For this review, take the finished solid that the model builds, in its own axes (mm). A direction names the side the tool comes from. Coordinates: 2 decimals unless noted, no trailing zeros. Write each loop counter-clockwise with the first axis right and the second up, starting at its lowest first coordinate (ties: lowest second). Pieces come first, ordered by that corner, then holes.
1) We need section A-A on z = 9.25. Write out the cut boundary in (x, y), then the cut area to 3 significant figures.
2) We need section B-B on y = -26.5. Write out the cut boundary in (x, z), then the cut area to 3 significant figures.
3) Mouldability with a two-part tool opening along Y and no side actions: class faces 3 (the face through (37, 55, 15)), 4 (the face through (42, 72.633, 12)), 5 (the face through (41, -66.524, 12)) as pulls with the +Y half, pulls with the -Y half, needs draft (parallel to the pull), parting line crosses it, or undercut.
4) To check wall thickness, follow line 1 along Y through (x, z) = (37, 18.5) (3 decimals); line 2 along Y through (x, z) = (32.5, 18.5); line 3 along Z through (x, y) = (31.5, -34). State the ranges of each line that lie inside material, in increasing order.
5) We need section C-C on x = 39. Write out the cut boundary in (y, z), then the cut area to 3 significant figures.
6) For faces 1 (the face through (32, -31, 3)), 2 (the face through (54.099, 2, 12)), list the 3-axis set-ups (+Z, -Z, +X, -X, +Y, -Y) from which the entire face can be reached by the end or side of a thin tool; tool diameter is ignored.
7) Insertion check: P1, Ø7, axis at x = 33.5, y = 52, coming from the +Z side; P2, Ø3, axis at x = 32.5, y = -28, coming from the +Z side. Each pin has a flat end and moves straight along its axis. Give the tip position at first contact, or say it passes through.
8) We need section D-D on z = 19.25. Write out the cut boundary in (x, y).
from build123d import *

# Parameters (mm, degrees)
F1_DEPTH = 25
F2_DEPTH = 3
F3_DEPTH = 15
F4_W     = 25
F4_H     = 139.1576522589
F5_DEPTH = 3


with BuildPart() as f1:
    # F0 (on Top) → F1 (new body)
    with BuildSketch(Plane.XY):
        with BuildLine():
            Line((54.0989699066, 72.6331850421), (29.0989699066, 72.6331850421))
            Line((29.0989699066, 72.6331850421), (29.0989699066, 67.49929167))
            ThreePointArc((29.0989699066, 67.49929167), (37.8737569223, 63.8034575596), (41.5, 54.9996834778))
            ThreePointArc((41.5, 54.9996834778), (37.8737569223, 46.195909396), (29.0989699066, 42.5000752856))
            Line((29.0989699066, 42.5000752856), (29.0989699066, 39.5786203772))
            ThreePointArc((29.0989699066, 39.5786203772), (37.8737569223, 35.8827862669), (41.5, 27.079012185))
            ThreePointArc((41.5, 27.079012185), (37.8737569223, 18.2752381032), (29.0989699066, 14.5794039929))
            Line((29.0989699066, 14.5794039929), (29.0989699066, 10.4122504635))
            ThreePointArc((29.0989699066, 10.4122504635), (37.8737569223, 6.7164163532), (41.5, -2.0873577287))
            ThreePointArc((41.5, -2.0873577287), (37.8737569223, -10.8911318105), (29.0989699066, -14.5869659208))
            Line((29.0989699066, -14.5869659208), (29.0989699066, -18.4864327763))
            ThreePointArc((29.0989699066, -18.4864327763), (37.8737569223, -22.1822668866), (41.5, -30.9860409684))
            ThreePointArc((41.5, -30.9860409684), (37.8737569223, -39.7898150502), (29.0989699066, -43.4856491606))
            Line((29.0989699066, -43.4856491606), (29.0989699066, -66.5244672167))
            Line((29.0989699066, -66.5244672167), (54.0989699066, -66.5244672167))
            Line((54.0989699066, -66.5244672167), (54.0989699066, 72.6331850421))
        make_face()
    extrude(amount=F1_DEPTH)



with BuildPart() as f2:
    # F0 (on Top) → F2 (new body)
    with BuildSketch(Plane.XY):
        with BuildLine():
            ThreePointArc((35.5, 54.9996834778), (33.6310530332, 59.5607521907), (29.0989699066, 61.4989299693))
            Line((29.0989699066, 61.4989299693), (29.0989699066, 48.5004369863))
            ThreePointArc((29.0989699066, 48.5004369863), (33.6310530332, 50.4386147649), (35.5, 54.9996834778))
        make_face()
    extrude(amount=F2_DEPTH)


with BuildPart() as f2b:
    # F0 (on Top) → F2, piece 2 (new body)
    with BuildSketch(Plane.XY):
        with BuildLine():
            ThreePointArc((35.5, 27.079012185), (33.6310530332, 31.6400808979), (29.0989699066, 33.5782586765))
            Line((29.0989699066, 33.5782586765), (29.0989699066, 20.5797656935))
            ThreePointArc((29.0989699066, 20.5797656935), (33.6310530332, 22.5179434721), (35.5, 27.079012185))
        make_face()
    extrude(amount=F2_DEPTH)


with BuildPart() as f2c:
    # F0 (on Top) → F2, piece 3 (new body)
    with BuildSketch(Plane.XY):
        with BuildLine():
            Line((29.0989699066, 4.4118887628), (29.0989699066, -8.5866042202))
            ThreePointArc((29.0989699066, -8.5866042202), (33.6310530332, -6.6484264416), (35.5, -2.0873577287))
            ThreePointArc((35.5, -2.0873577287), (33.6310530332, 2.4737109842), (29.0989699066, 4.4118887628))
        make_face()
    extrude(amount=F2_DEPTH)


with BuildPart() as f2d:
    # F0 (on Top) → F2, piece 4 (new body)
    with BuildSketch(Plane.XY):
        with BuildLine():
            Line((29.0989699066, -24.4867944769), (29.0989699066, -37.4852874599))
            ThreePointArc((29.0989699066, -37.4852874599), (33.6310530332, -35.5471096813), (35.5, -30.9860409684))
            ThreePointArc((35.5, -30.9860409684), (33.6310530332, -26.4249722555), (29.0989699066, -24.4867944769))
        make_face()
    extrude(amount=F2_DEPTH)


with BuildPart() as f1_1:
    add(f1.part)

    add(f2.part)  # F3 merges F2

    add(f2b.part)  # F3 merges F2b

    add(f2c.part)  # F3 merges F2c

    add(f2d.part)  # F3 merges F2d
    # F0 (on Top) → F3 (join)
    with BuildSketch(Plane.XY):
        with BuildLine():
            ThreePointArc((41.5, 54.9996834778), (37.8737569223, 63.8034575596), (29.0989699066, 67.49929167))
            Line((29.0989699066, 67.49929167), (29.0989699066, 61.4989299693))
            ThreePointArc((29.0989699066, 61.4989299693), (33.6310530332, 59.5607521907), (35.5, 54.9996834778))
            ThreePointArc((35.5, 54.9996834778), (33.6310530332, 50.4386147649), (29.0989699066, 48.5004369863))
            Line((29.0989699066, 48.5004369863), (29.0989699066, 42.5000752856))
            ThreePointArc((29.0989699066, 42.5000752856), (37.8737569223, 46.195909396), (41.5, 54.9996834778))
        make_face()
        with BuildLine():
            ThreePointArc((41.5, 27.079012185), (37.8737569223, 35.8827862669), (29.0989699066, 39.5786203772))
            Line((29.0989699066, 39.5786203772), (29.0989699066, 33.5782586765))
            ThreePointArc((29.0989699066, 33.5782586765), (33.6310530332, 31.6400808979), (35.5, 27.079012185))
            ThreePointArc((35.5, 27.079012185), (33.6310530332, 22.5179434721), (29.0989699066, 20.5797656935))
            Line((29.0989699066, 20.5797656935), (29.0989699066, 14.5794039929))
            ThreePointArc((29.0989699066, 14.5794039929), (37.8737569223, 18.2752381032), (41.5, 27.079012185))
        make_face()
        with BuildLine():
            Line((29.0989699066, -8.5866042202), (29.0989699066, -14.5869659208))
            ThreePointArc((29.0989699066, -14.5869659208), (37.8737569223, -10.8911318105), (41.5, -2.0873577287))
            ThreePointArc((41.5, -2.0873577287), (37.8737569223, 6.7164163532), (29.0989699066, 10.4122504635))
            Line((29.0989699066, 10.4122504635), (29.0989699066, 4.4118887628))
            ThreePointArc((29.0989699066, 4.4118887628), (33.6310530332, 2.4737109842), (35.5, -2.0873577287))
            ThreePointArc((35.5, -2.0873577287), (33.6310530332, -6.6484264416), (29.0989699066, -8.5866042202))
        make_face()
        with BuildLine():
            Line((29.0989699066, -37.4852874599), (29.0989699066, -43.4856491606))
            ThreePointArc((29.0989699066, -43.4856491606), (37.8737569223, -39.7898150502), (41.5, -30.9860409684))
            ThreePointArc((41.5, -30.9860409684), (37.8737569223, -22.1822668866), (29.0989699066, -18.4864327763))
            Line((29.0989699066, -18.4864327763), (29.0989699066, -24.4867944769))
            ThreePointArc((29.0989699066, -24.4867944769), (33.6310530332, -26.4249722555), (35.5, -30.9860409684))
            ThreePointArc((35.5, -30.9860409684), (33.6310530332, -35.5471096813), (29.0989699066, -37.4852874599))
        make_face()
    extrude(amount=F3_DEPTH)

    # F4 (on face) → F5 (join)
    with BuildSketch(Plane(origin=(0, 0, 0), x_dir=(1, 0, 0), z_dir=(0, 0, -1))):
        with Locations((41.5989699066, -3.0543589127)):
            Rectangle(F4_W, F4_H)
    extrude(amount=-F5_DEPTH)


solid = f1_1.part
Result:
1. outline: (29.1, -66.52) - (54.1, -66.52) - (54.1, 72.63) - (29.1, 72.63) - (29.1, 61.5) arc R6.5 cw to (29.1, 48.5) - (29.1, 33.58) arc R6.5 cw to (29.1, 20.58) - (29.1, 4.41) arc R6.5 cw to (29.1, -8.59) - (29.1, -24.49) arc R6.5 cw to (29.1, -37.49) - close
1. area: 3,220 mm2
2. outline: (29.1, 0) - (54.1, 0) - (54.1, 25) - (40.67, 25) - (40.67, 15) - (33.7, 15) - (33.7, 3) - (29.1, 3) - close
2. area: 454 mm2
3. face 3: undercut
3. face 4: pulls with the +Y half
3. face 5: pulls with the -Y half
4. line 1: y = -66.524 to -40.591, -21.381 to -11.692, 7.517 to 17.474, 36.684 to 45.395, 64.604 to 72.633
4. line 2: y = -66.52 to -42.99, -18.99 to -14.09, 9.91 to 15.08, 39.08 to 43, 67 to 72.63
4. line 3: z = 0 to 3
5. outline: (-66.52, 0) - (72.63, 0) - (72.63, 25) - (62.5, 25) - (62.5, 15) - (47.5, 15) - (47.5, 25) - (34.58, 25) - (34.58, 15) - (19.58, 15) - (19.58, 25) - (5.41, 25) - (5.41, 15) - (-9.59, 15) - (-9.59, 25) - (-23.49, 25) - (-23.49, 15) - (-38.49, 15) - (-38.49, 25) - (-66.52, 25) - close
5. area: 2,880 mm2
6. face 1: +Z, -X
6. face 2: +Z, -Z, +X, +Y, -Y
7. P1: stops at z = 15
7. P2: stops at z = 3
8. outline: (29.1, -66.52) - (54.1, -66.52) - (54.1, 72.63) - (29.1, 72.63) - (29.1, 67.5) arc R12.5 cw to (29.1, 42.5) - (29.1, 39.58) arc R12.5 cw to (29.1, 14.58) - (29.1, 10.41) arc R12.5 cw to (29.1, -14.59) - (29.1, -18.49) arc R12.5 cw to (29.1, -43.49) - close
